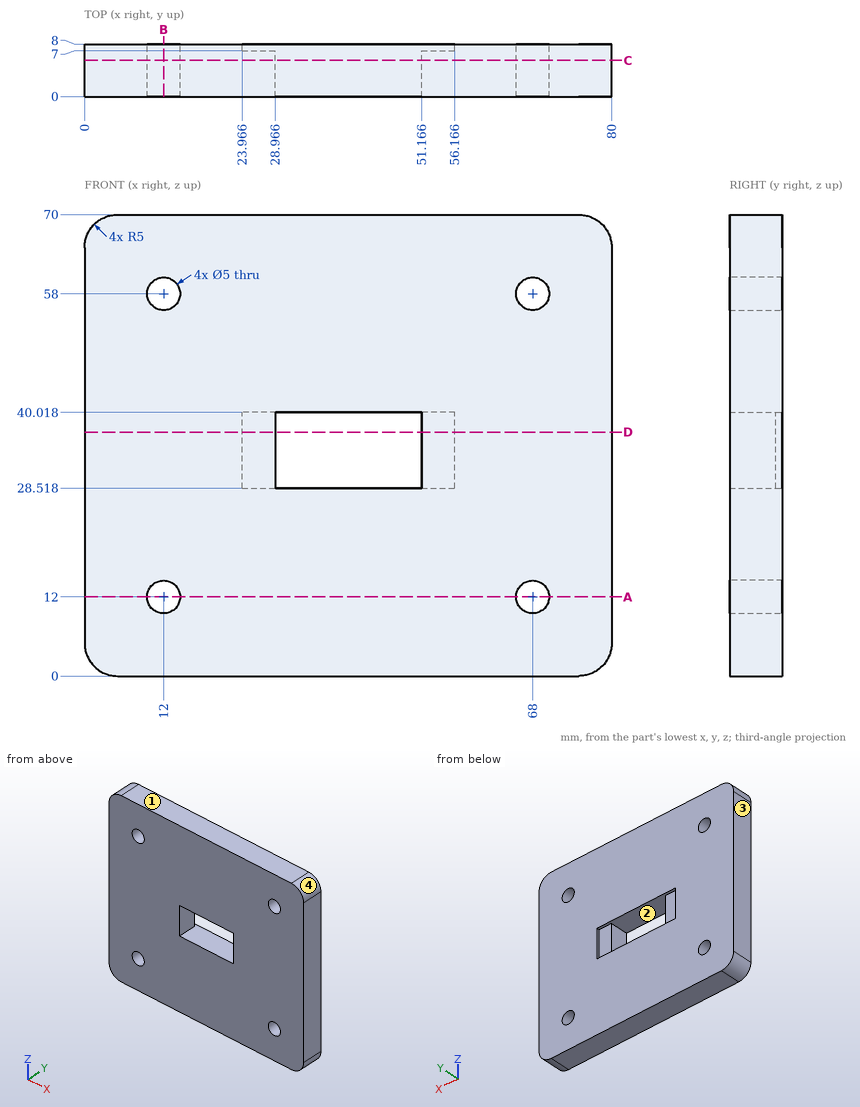
Print and shaded views of the part. All mm, measured from the part's lowest x, y and z. Coordinates: 2 decimals unless noted, no trailing zeros. Loops run counter-clockwise (first coordinate to the right, second up) from the corner with the lowest first, then second, coordinate; pieces in that order, holes last. Notation, with made-up numbers: (-14.75, -32) - (-10.75, -32) arc R16 cw to (-10.75, -4) - close; hole circle Ø4 at (-21, 7.5). An arc over 180 degrees is marked (long way). Use one line per item in the form item = value. Start each with the question number.
1) Two-plate mould, pull along X, no slides. Class the marked faces 1, 2, 3 and 4: +X half, -X half, draft (parallel to the pull), parting line (faces both ways), or undercut.
2) Band-saw the part on B-B (x = 12). Give the cut face in (y, z), and give its area (3 significant figures).
3) Band-saw the part on A-A (z = 12). Give the cut face in (x, y).
4) Flat gauge pins, fed straight in: pin 1 (6 mm diameter, centred on x = 12, z = 12, fed in from +Y); pin 2 (2.5 mm diameter, centred on x = 53, z = 35, fed in from +Y). Where does each tip first touch, or does it go through?
5) Band-saw the part on C-C (y = 5.5). Give the cut face in (x, z).
6) Band-saw the part on D-D (z = 37). Give the cut face in (x, y).
7) Drill centre lines: L1, parallel to X at y = 5.5, z = 58; L2, parallel to Z at x = 68, y = 3; L3, parallel to X at y = 0.5, z = 29.5. Where is each one in solid material? Low to high. Write a range as from..to.
Check values:
q1.face_1 = draft
q1.face_2 = undercut
q1.face_3 = -X half
q1.face_4 = +X half
q2.outline = (0, 0) - (8, 0) - (8, 9.5) - (0, 9.5) - close; (0, 14.5) - (8, 14.5) - (8, 55.5) - (0, 55.5) - close; (0, 60.5) - (8, 60.5) - (8, 70) - (0, 70) - close
q2.area = 480 mm2
q3.outline = (0, 0) - (9.5, 0) - (9.5, 8) - (0, 8) - close; (14.5, 0) - (65.5, 0) - (65.5, 8) - (14.5, 8) - close; (70.5, 0) - (80, 0) - (80, 8) - (70.5, 8) - close
q4.pin_1 = 8
q4.pin_2 = 7
q5.outline = (0, 5) arc R5 ccw to (5, 0) - (75, 0) arc R5 ccw to (80, 5) - (80, 65) arc R5 ccw to (75, 70) - (5, 70) arc R5 ccw to (0, 65) - close; hole circle Ø5 at (12, 12); hole circle Ø5 at (12, 58); hole (28.97, 28.52) - (51.17, 28.52) - (51.17, 40.02) - (28.97, 40.02) - close; hole circle Ø5 at (68, 12); hole circle Ø5 at (68, 58)
q6.outline = (0, 0) - (28.97, 0) - (28.97, 7) - (23.97, 7) - (23.97, 8) - (0, 8) - close; (51.17, 0) - (80, 0) - (80, 8) - (56.17, 8) - (56.17, 7) - (51.17, 7) - close
q7.L1 = 0..9.5, 14.5..65.5, 70.5..80
q7.L2 = 0..9.5, 14.5..55.5, 60.5..70
q7.L3 = 0..28.97, 51.17..80
